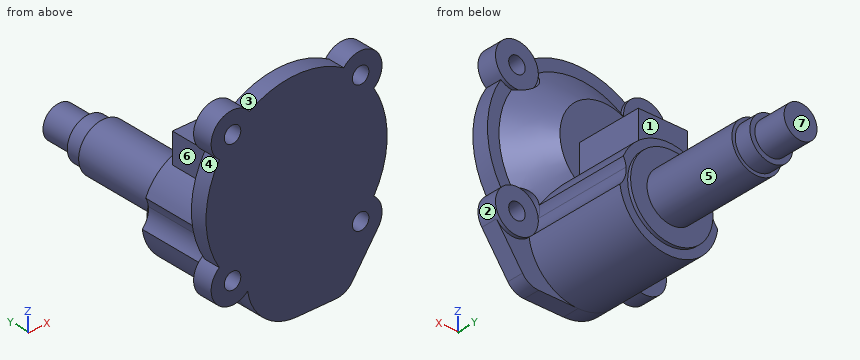
from build123d import *

# Parameters (mm, degrees)
SKETCH1_R               = 27.5
BOSS_EXTRUDE1_DEPTH     = 5
SKETCH3_R               = 2.5
CUT_EXTRUDE1_DEPTH      = 6
CUT_EXTRUDE1_DEPTH_BACK = 1
SKETCH3_3_R             = 6.5
SKETCH3_3_R_2           = 2.5
BOSS_EXTRUDE2_DEPTH     = 6
SKETCH5_R               = 6.5
CUT_EXTRUDE2_DEPTH      = 6
BOSS_EXTRUDE3_DEPTH     = 31
SKETCH7_R               = 12.5
BOSS_EXTRUDE4_DEPTH     = 1
SKETCH8_R               = 7.5
BOSS_EXTRUDE5_DEPTH     = 29
SKETCH9_R               = 6.5
BOSS_EXTRUDE6_DEPTH     = 5
SKETCH10_R              = 5
BOSS_EXTRUDE7_DEPTH     = 10
BOSS_EXTRUDE11_DEPTH    = 5
SKETCH13_W              = 15
SKETCH13_H              = 11.899909518
BOSS_EXTRUDE12_DEPTH    = 20


with BuildPart() as part:
    # Sketch1 → Boss-Extrude1 (new body)
    with BuildSketch(Plane(origin=(0, 0, 0), x_dir=(1, 0, 0), z_dir=(0, 1, 0))):
        Circle(SKETCH1_R)
    extrude(amount=BOSS_EXTRUDE1_DEPTH)

    # Sketch3 → Cut-Extrude1 (cut, two sides)
    with BuildSketch(Plane(origin=(0, 0, 0), x_dir=(1, 0, 0), z_dir=(0, 1, 0))) as cut_extrude1_sk:
        with Locations((-19.445436483, -19.445436483)):
            Circle(SKETCH3_R)
        with Locations((-19.445436483, 19.445436483)):
            Circle(SKETCH3_R)
        with Locations((19.445436483, 19.445436483)):
            Circle(SKETCH3_R)
        with Locations((19.445436483, -19.445436483)):
            Circle(SKETCH3_R)
    extrude(amount=CUT_EXTRUDE1_DEPTH, mode=Mode.SUBTRACT)
    extrude(cut_extrude1_sk.sketch, amount=-CUT_EXTRUDE1_DEPTH_BACK, mode=Mode.SUBTRACT)

    # Sketch3<3> → Boss-Extrude2 (add)
    with BuildSketch(Plane(origin=(0, 0, 0), x_dir=(1, 0, 0), z_dir=(0, 1, 0))):
        with Locations((-19.445436483, -19.445436483)):
            Circle(SKETCH3_3_R)
        with Locations((-19.445436483, -19.445436483)):
            Circle(SKETCH3_3_R_2, mode=Mode.SUBTRACT)
        with Locations((-19.445436483, 19.445436483)):
            Circle(SKETCH3_3_R)
        with Locations((-19.445436483, 19.445436483)):
            Circle(SKETCH3_3_R_2, mode=Mode.SUBTRACT)
        with Locations((19.445436483, 19.445436483)):
            Circle(SKETCH3_3_R)
        with Locations((19.445436483, 19.445436483)):
            Circle(SKETCH3_3_R_2, mode=Mode.SUBTRACT)
        with Locations((19.445436483, -19.445436483)):
            Circle(SKETCH3_3_R)
        with Locations((19.445436483, -19.445436483)):
            Circle(SKETCH3_3_R_2, mode=Mode.SUBTRACT)
    extrude(amount=BOSS_EXTRUDE2_DEPTH)

    # Sketch4 → Revolve1 (revolve)
    with BuildSketch(Plane.XY):
        Polygon((0, 5), (-24, 5), (-13.5, 14), (0, 14), align=None)
    revolve(axis=Axis((0, 14, 0), (0, -1, 0)))

    # Sketch5 → Cut-Extrude2 (cut)
    with BuildSketch(Plane(origin=(0, 6, 0), x_dir=(1, 0, 0), z_dir=(0, 1, 0))):
        with Locations((19.445436483, -19.445436483)):
            Circle(SKETCH5_R)
        with Locations((19.445436483, 19.445436483)):
            Circle(SKETCH5_R)
        with Locations((-19.445436483, 19.445436483)):
            Circle(SKETCH5_R)
        with Locations((-19.445436483, -19.445436483)):
            Circle(SKETCH5_R)
    extrude(amount=CUT_EXTRUDE2_DEPTH, mode=Mode.SUBTRACT)

    # Sketch6 → Boss-Extrude3 (add)
    with BuildSketch(Plane(origin=(0, 5, 0), x_dir=(1, 0, 0), z_dir=(0, 1, 0))):
        with BuildLine():
            ThreePointArc((14.859059475, 24.051426706), (0, 37), (-14.859059475, 24.051426706))
            ThreePointArc((-14.859059475, 24.051426706), (-13.323926947, 21.631099084), (-12.9789923, 18.78581566))
            ThreePointArc((-12.9789923, 18.78581566), (-13.26319033, 17.437992209), (-13.825025584, 16.180320661))
            ThreePointArc((-13.825025584, 16.180320661), (0, 7), (13.825025584, 16.180320661))
            ThreePointArc((13.825025584, 16.180320661), (13.26319033, 17.437992209), (12.9789923, 18.78581566))
            ThreePointArc((12.9789923, 18.78581566), (13.323926947, 21.631099084), (14.859059475, 24.051426706))
        make_face()
    extrude(amount=BOSS_EXTRUDE3_DEPTH)

    # Sketch7 → Boss-Extrude4 (add)
    with BuildSketch(Plane(origin=(0, 36, 0), x_dir=(1, 0, 0), z_dir=(0, 1, 0))):
        with Locations((0, 22)):
            Circle(SKETCH7_R)
    extrude(amount=BOSS_EXTRUDE4_DEPTH)

    # Sketch8 → Boss-Extrude5 (add)
    with BuildSketch(Plane(origin=(0, 37, 0), x_dir=(1, 0, 0), z_dir=(0, 1, 0))):
        with Locations((0, 22)):
            Circle(SKETCH8_R)
    extrude(amount=BOSS_EXTRUDE5_DEPTH)

    # Sketch9 → Boss-Extrude6 (add)
    with BuildSketch(Plane(origin=(0, 66, 0), x_dir=(1, 0, 0), z_dir=(0, 1, 0))):
        with Locations((0, 22)):
            Circle(SKETCH9_R)
    extrude(amount=BOSS_EXTRUDE6_DEPTH)

    # Sketch10 → Boss-Extrude7 (add)
    with BuildSketch(Plane(origin=(0, 71, 0), x_dir=(1, 0, 0), z_dir=(0, 1, 0))):
        with Locations((0, 22)):
            Circle(SKETCH10_R)
    extrude(amount=BOSS_EXTRUDE7_DEPTH)

    # Sketch12 → Boss-Extrude11 (add)
    with BuildSketch(Plane(origin=(0, 0, 0), x_dir=(1, 0, 0), z_dir=(0, 1, 0))):
        with BuildLine():
            Line((24.769924771, 23.173683319), (16.880143567, 34.441458618))
            ThreePointArc((16.880143567, 34.441458618), (14.735722981, 36.322064999), (11.965231301, 37))
            Line((11.965231301, 37), (0, 37))
            ThreePointArc((0, 37), (-9.854658782, 33.30865599), (-14.859059475, 24.051426706))
            ThreePointArc((-14.859059475, 24.051426706), (-14.589838885, 23.766683059), (-14.338266086, 23.466233734))
            ThreePointArc((-14.338266086, 23.466233734), (0, 27.5), (14.338266086, 23.466233734))
            ThreePointArc((14.338266086, 23.466233734), (14.589838885, 23.766683059), (14.859059475, 24.051426706))
            ThreePointArc((14.859059475, 24.051426706), (20.018856424, 25.920093969), (24.769924771, 23.173683319))
        make_face()
    extrude(amount=BOSS_EXTRUDE11_DEPTH)

    # Sketch13 → Boss-Extrude12 (add)
    with BuildSketch(Plane(origin=(0, 14, 0), x_dir=(1, 0, 0), z_dir=(0, 1, 0))):
        with Locations((0, 5.949954759)):
            Rectangle(SKETCH13_W, SKETCH13_H)
    extrude(amount=BOSS_EXTRUDE12_DEPTH)


solid = part.part
Geometry check sheet. Reference: the model listing, model coordinates, mm. Face numbers are marked on the shaded views. A direction names the side the tool comes from. Give positions to 0.01 mm unless a question says otherwise; leave off trailing zeros. Loops run counter-clockwise (first coordinate to the right, second up) from the corner with the lowest first, then second, coordinate; pieces in that order, holes last.
(1) Section check A-A on y = 26.5. Record the cut outline in (x, z), then the cut area to 3 significant figures.
From the geometry:
outline: (-14.86, -24.05) arc R15 ccw to (14.86, -24.05) arc R6.5 cw to (13.83, -16.18) arc R15 ccw to (7.5, -9.01) - (7.5, 0) - (-7.5, 0) - (-7.5, -9.01) arc R15 ccw to (-13.83, -16.18) arc R6.5 cw to start
area: 801 mm2
(2) Release check for a two-part mould opening along Z. For the marked faces 1, 2, 3 and 4 record: released by +Z, released by -Z, zero draft, split by the parting line, or undercut.
From the geometry:
face 1: zero draft
face 2: undercut
face 3: released by +Z
face 4: undercut
(3) Section check C-C on z = -31.5. Record the cut outline in (x, y).
From the geometry:
outline: (-11.61, 0) - (18.94, 0) - (18.94, 5) - (11.61, 5) - (11.61, 36) - (8.12, 36) - (8.12, 37) - (-8.12, 37) - (-8.12, 36) - (-11.61, 36) - close
(4) Set-up check for the marked faces 5, 6 and 7: record each of +Z, -Z, +X, -X, +Y, -Y from which the full face is reachable in a straight line by a thin tool's end or side.
From the geometry:
face 5: +Y
face 6: +Z, -X, +Y
face 7: +Z, -Z, +X, -X, +Y
(5) Depth check by flat-ended pin: pin 1 Ø1.5 at (x, z) = (-13, 7) entering from +Y; pin 2 Ø6 at (y, z) = (37.5, -6) entering from +X; pin 3 Ø14.5 at (x, z) = (-19.5, -20.5) entering from +Y. Enter the tip coordinate at first touch or a pass-through.
From the geometry:
pin 1: stops at y = 13.56
pin 2: stops at x = 6.74
pin 3: stops at y = 37
(6) Thickness scan on L1, parallel to Y at x = 20, z = -29; L2, parallel to Y at x = -1, z = -32; L3, parallel to X at y = 25, z = -1. Record the ranges inside material, lowest first.
From the geometry:
L1: y = 0 to 5
L2: y = 0 to 37
L3: x = -7.5 to 7.5
(7) Section check D-D on y = 60.5. Record the cut outline in (x, z).
From the geometry:
outline: circle Ø15 at (0, -22)
